```python
from build123d import *

# Parameters (mm, degrees)
CUT_EXTRUDE1_DEPTH = 10
SKETCH4_W          = 10
SKETCH4_H          = 10
CUT_EXTRUDE2_DEPTH = 4


with BuildPart() as part:
    # Sketch1 → Revolve1 (revolve)
    with BuildSketch(Plane.XY, mode=Mode.PRIVATE) as revolve1_sk:
        Polygon((2.5, 0), (12.5, 0), (12.5, 4), (6, 6), (2.5, 6), align=None)
    revolve(revolve1_sk.sketch.rotate(Axis((0, 6, 0), (0, -1, 0)), 180), axis=Axis((0, 6, 0), (0, -1, 0)))

    # Sketch2 → Cut-Extrude1 (cut)
    with BuildSketch(Plane.XZ):
        with BuildLine():
            Line((-0.75, 13), (0.75, 13))
            ThreePointArc((0.75, 13), (1.25, 12.5), (0.75, 12))
            Line((0.75, 12), (-0.75, 12))
            ThreePointArc((-0.75, 12), (-1.25, 12.5), (-0.75, 13))
        make_face()
        with BuildLine():
            Line((3.741492398, 12.472519178), (5.151031329, 11.959488963))
            ThreePointArc((5.151031329, 11.959488963), (5.449867568, 11.318632581), (4.809011185, 11.019796342))
            Line((4.809011185, 11.019796342), (3.399472254, 11.532826557))
            ThreePointArc((3.399472254, 11.532826557), (3.100636016, 12.173682939), (3.741492398, 12.472519178))
        make_face()
        with BuildLine():
            Line((7.781705594, 10.440668468), (8.930772258, 9.476487053))
            ThreePointArc((8.930772258, 9.476487053), (8.992400675, 8.772071027), (8.287984649, 8.71044261))
            Line((8.287984649, 8.71044261), (7.138917984, 9.674624025))
            ThreePointArc((7.138917984, 9.674624025), (7.077289567, 10.379040051), (7.781705594, 10.440668468))
        make_face()
        with BuildLine():
            Line((10.883330249, 7.149519053), (11.633330249, 5.850480947))
            ThreePointArc((11.633330249, 5.850480947), (11.450317547, 5.167468245), (10.767304845, 5.350480947))
            Line((10.767304845, 5.350480947), (10.017304845, 6.649519053))
            ThreePointArc((10.017304845, 6.649519053), (10.200317547, 7.332531755), (10.883330249, 7.149519053))
        make_face()
        with BuildLine():
            Line((12.672264656, 2.996032124), (12.932736922, 1.518820495))
            ThreePointArc((12.932736922, 1.518820495), (12.527157135, 0.93959253), (11.947929169, 1.345172317))
            Line((11.947929169, 1.345172317), (11.687456903, 2.822383947))
            ThreePointArc((11.687456903, 2.822383947), (12.093036691, 3.401611912), (12.672264656, 2.996032124))
        make_face()
        with BuildLine():
            Line((12.932736922, -1.518820495), (12.672264656, -2.996032124))
            ThreePointArc((12.672264656, -2.996032124), (12.093036691, -3.401611912), (11.687456903, -2.822383947))
            Line((11.687456903, -2.822383947), (11.947929169, -1.345172317))
            ThreePointArc((11.947929169, -1.345172317), (12.527157135, -0.93959253), (12.932736922, -1.518820495))
        make_face()
        with BuildLine():
            Line((11.633330249, -5.850480947), (10.883330249, -7.149519053))
            ThreePointArc((10.883330249, -7.149519053), (10.200317547, -7.332531755), (10.017304845, -6.649519053))
            Line((10.017304845, -6.649519053), (10.767304845, -5.350480947))
            ThreePointArc((10.767304845, -5.350480947), (11.450317547, -5.167468245), (11.633330249, -5.850480947))
        make_face()
        with BuildLine():
            Line((8.930772258, -9.476487053), (7.781705594, -10.440668468))
            ThreePointArc((7.781705594, -10.440668468), (7.077289567, -10.379040051), (7.138917984, -9.674624025))
            Line((7.138917984, -9.674624025), (8.287984649, -8.71044261))
            ThreePointArc((8.287984649, -8.71044261), (8.992400675, -8.772071027), (8.930772258, -9.476487053))
        make_face()
        with BuildLine():
            Line((5.151031329, -11.959488963), (3.741492398, -12.472519178))
            ThreePointArc((3.741492398, -12.472519178), (3.100636016, -12.173682939), (3.399472254, -11.532826557))
            Line((3.399472254, -11.532826557), (4.809011185, -11.019796342))
            ThreePointArc((4.809011185, -11.019796342), (5.449867568, -11.318632581), (5.151031329, -11.959488963))
        make_face()
        with BuildLine():
            Line((0.75, -13), (-0.75, -13))
            ThreePointArc((-0.75, -13), (-1.25, -12.5), (-0.75, -12))
            Line((-0.75, -12), (0.75, -12))
            ThreePointArc((0.75, -12), (1.25, -12.5), (0.75, -13))
        make_face()
        with BuildLine():
            Line((-3.741492398, -12.472519178), (-5.151031329, -11.959488963))
            ThreePointArc((-5.151031329, -11.959488963), (-5.449867568, -11.318632581), (-4.809011185, -11.019796342))
            Line((-4.809011185, -11.019796342), (-3.399472254, -11.532826557))
            ThreePointArc((-3.399472254, -11.532826557), (-3.100636016, -12.173682939), (-3.741492398, -12.472519178))
        make_face()
        with BuildLine():
            Line((-7.781705594, -10.440668468), (-8.930772258, -9.476487053))
            ThreePointArc((-8.930772258, -9.476487053), (-8.992400675, -8.772071027), (-8.287984649, -8.71044261))
            Line((-8.287984649, -8.71044261), (-7.138917984, -9.674624025))
            ThreePointArc((-7.138917984, -9.674624025), (-7.077289567, -10.379040051), (-7.781705594, -10.440668468))
        make_face()
        with BuildLine():
            Line((-10.883330249, -7.149519053), (-11.633330249, -5.850480947))
            ThreePointArc((-11.633330249, -5.850480947), (-11.450317547, -5.167468245), (-10.767304845, -5.350480947))
            Line((-10.767304845, -5.350480947), (-10.017304845, -6.649519053))
            ThreePointArc((-10.017304845, -6.649519053), (-10.200317547, -7.332531755), (-10.883330249, -7.149519053))
        make_face()
        with BuildLine():
            Line((-12.672264656, -2.996032124), (-12.932736922, -1.518820495))
            ThreePointArc((-12.932736922, -1.518820495), (-12.527157135, -0.93959253), (-11.947929169, -1.345172317))
            Line((-11.947929169, -1.345172317), (-11.687456903, -2.822383947))
            ThreePointArc((-11.687456903, -2.822383947), (-12.093036691, -3.401611912), (-12.672264656, -2.996032124))
        make_face()
        with BuildLine():
            Line((-12.932736922, 1.518820495), (-12.672264656, 2.996032124))
            ThreePointArc((-12.672264656, 2.996032124), (-12.093036691, 3.401611912), (-11.687456903, 2.822383947))
            Line((-11.687456903, 2.822383947), (-11.947929169, 1.345172317))
            ThreePointArc((-11.947929169, 1.345172317), (-12.527157135, 0.93959253), (-12.932736922, 1.518820495))
        make_face()
        with BuildLine():
            Line((-11.633330249, 5.850480947), (-10.883330249, 7.149519053))
            ThreePointArc((-10.883330249, 7.149519053), (-10.200317547, 7.332531755), (-10.017304845, 6.649519053))
            Line((-10.017304845, 6.649519053), (-10.767304845, 5.350480947))
            ThreePointArc((-10.767304845, 5.350480947), (-11.450317547, 5.167468245), (-11.633330249, 5.850480947))
        make_face()
        with BuildLine():
            Line((-8.930772258, 9.476487053), (-7.781705594, 10.440668468))
            ThreePointArc((-7.781705594, 10.440668468), (-7.077289567, 10.379040051), (-7.138917984, 9.674624025))
            Line((-7.138917984, 9.674624025), (-8.287984649, 8.71044261))
            ThreePointArc((-8.287984649, 8.71044261), (-8.992400675, 8.772071027), (-8.930772258, 9.476487053))
        make_face()
        with BuildLine():
            Line((-5.151031329, 11.959488963), (-3.741492398, 12.472519178))
            ThreePointArc((-3.741492398, 12.472519178), (-3.100636016, 12.173682939), (-3.399472254, 11.532826557))
            Line((-3.399472254, 11.532826557), (-4.809011185, 11.019796342))
            ThreePointArc((-4.809011185, 11.019796342), (-5.449867568, 11.318632581), (-5.151031329, 11.959488963))
        make_face()
    extrude(amount=-CUT_EXTRUDE1_DEPTH, mode=Mode.SUBTRACT)

    # Sketch4 → Cut-Extrude2 (cut)
    with BuildSketch(Plane(origin=(0, 0, 0), x_dir=(1, 0, 0), z_dir=(0, 1, 0))):
        Rectangle(SKETCH4_W, SKETCH4_H)
    extrude(amount=CUT_EXTRUDE2_DEPTH, mode=Mode.SUBTRACT)


solid = part.part
```
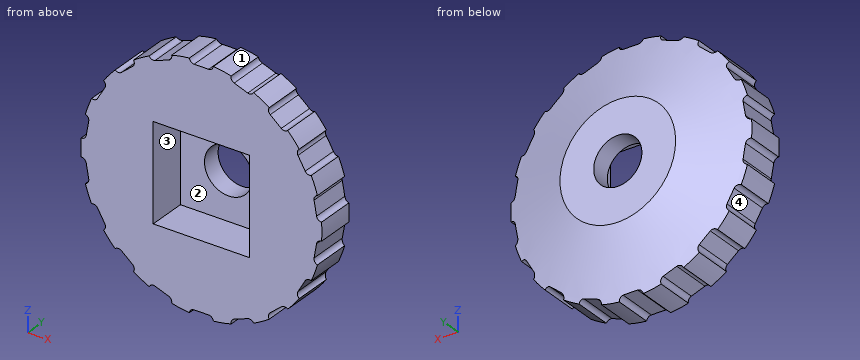
For this review, take the finished solid that the model builds, in its own axes (mm). Face numbers are marked on the shaded views. Give positions to 0.01 mm unless a question says otherwise; leave off trailing zeros. Write each loop counter-clockwise with the first axis right and the second up, starting at its lowest first coordinate (ties: lowest second). Pieces come first, ordered by that corner, then holes. Notation, with made-up numbers: M 69.25,67.25 L 78.25,67.25 A18 ccw 78.25,80.25 Z; hole C 68.25,45.25 d5. An arc over 180 degrees is marked long. Answer as a JSON object with one key per item and string values. Group by question number.
Item 1: Consider section B-B on x = 0. Write out the cut boundary in (y, z), plus the area to 3 significant figures.
Item 2: Consider section C-C on y = 4.75. Write out the cut boundary in (x, z) (1 decimal).
Item 3: Draft analysis for pull direction X (two halves, no side actions). For the marked faces 1, 2, 3 and 4, state which applies: +X half, -X half, draft (parallel to the pull), parting line (faces both ways), or undercut.
Item 4: Consider section A-A on z = 0. Write out the cut boundary in (x, y), plus the area to 3 significant figures.
Item 5: For probe 1 along X at (y, z) = (1.5, 4.5); probe 2 along X at (y, z) = (1, -1.5); probe 3 along Z at (x, y) = (3, 2.75), list the stretches that pass through material, from the lowest coordinate up. Write a range as [from, to].
Item 6: For pin 1 Ø2 at (y, z) = (2.5, 1.5) entering from +X; pin 2 Ø6 at (x, z) = (0, 0) entering from -Y; pin 3 Ø1.2 at (y, z) = (3, -1.5) entering from -X, all flat-tipped, find the tip position at first contact; note any pin that passes through.
Check result:
{
 "1": {"outline": "M 0,-12 L 4.15,-12 L 6,-6 L 6,-2.5 L 4,-2.5 L 4,-5 L 0,-5 Z; M 0,5 L 4,5 L 4,2.5 L 6,2.5 L 6,6 L 4.15,12 L 0,12 Z", "area": "82.9 mm^2"},
 "2": {"outline": "C 0,0 d20.1; hole C 0,0 d5"},
 "3": {"face 1": "+X half", "face 2": "undercut", "face 3": "undercut", "face 4": "-X half"},
 "4": {"outline": "M -12.5,0 L -5,0 L -5,4 L -2.5,4 L -2.5,6 L -6,6 L -12.5,4 Z; M 2.5,4 L 5,4 L 5,0 L 12.5,0 L 12.5,4 L 6,6 L 2.5,6 Z", "area": "87.0 mm^2"},
 "5": {"probe 1": "x = [-11.66, -5], [5, 11.66]", "probe 2": "x = [-11.92, -5], [5, 11.92]", "probe 3": "z = [-12.13, -5], [5, 12.13]"},
 "6": {"pin 1": "stops at x = 12.49", "pin 2": "stops at y = 4", "pin 3": "stops at x = -12.47"}
}
